Here's how the part is built. I have some questions about the finished solid (model axes, mm). A direction names the side the tool comes from. Round coordinates to 2 decimals unless told otherwise and drop trailing zeros. Order: outer loops, then holes, each group sorted by start corner. A loop starts at its lowest first (then second) coordinate and runs counter-clockwise, first axis right, second up. Notation, with made-up numbers: M 55,5.25 L 62,5.25 A18 ccw 62,23.25 Z; hole C 24.25,4 d8. An arc over 180 degrees is marked long. Use one line per item in the form item = value. Start each with the question number.
```python
from build123d import *

# Parameters (mm, degrees)
SKETCH1_W           = 10
SKETCH1_H           = 12
SKETCH1_R           = 0.7
BOSS_EXTRUDE1_DEPTH = 9
BOSS_EXTRUDE2_DEPTH = 10
BOSS_EXTRUDE4_DEPTH = 0.7
BOSS_EXTRUDE5_DEPTH = 10
FILLET1_R           = 1
FILLET2_R           = 0.25


with BuildPart() as part:
    # Sketch1 → Boss-Extrude1 (new body)
    # profile 1 of 3: a face of its own
    with BuildSketch(Plane.XY):
        Rectangle(SKETCH1_W, SKETCH1_H)
        with Locations((0, 4.5)):
            Circle(SKETCH1_R, mode=Mode.SUBTRACT)
        with Locations((0, -4.5)):
            Circle(SKETCH1_R, mode=Mode.SUBTRACT)
    # profile 2 of 3: a face of its own
    with BuildSketch(Plane.XY):
        with Locations((0, -4.5)):
            Circle(SKETCH1_R)
    # profile 3 of 3: a face of its own
    with BuildSketch(Plane.XY):
        with Locations((0, 4.5)):
            Circle(SKETCH1_R)
    extrude(amount=-BOSS_EXTRUDE1_DEPTH)

    # Sketch2 → Boss-Extrude2 (add)
    with BuildSketch(Plane(origin=(5, 0, 0), x_dir=(0, 0, -1), z_dir=(1, 0, 0))):
        with BuildLine():
            Line((3.4, 5.949159605), (0, 4.043822449))
            Line((0, 4.043822449), (0, -4.043822449))
            Line((0, -4.043822449), (3.4, -5.949159605))
            ThreePointArc((3.4, -5.949159605), (3.561551285, -5.976772876), (3.723791265, -6))
            Line((3.723791265, -6), (5.276208735, -6))
            ThreePointArc((5.276208735, -6), (5.438448715, -5.976772876), (5.6, -5.949159605))
            Line((5.6, -5.949159605), (9, -4.043822449))
            Line((9, -4.043822449), (9, 4.043822449))
            Line((9, 4.043822449), (5.6, 5.949159605))
            ThreePointArc((5.6, 5.949159605), (5.438448715, 5.976772876), (5.276208735, 6))
            Line((5.276208735, 6), (3.723791265, 6))
            ThreePointArc((3.723791265, 6), (3.561551285, 5.976772876), (3.4, 5.949159605))
        make_face()
        with BuildLine():
            ThreePointArc((5.276208735, 6), (4.5, 6.05), (3.723791265, 6))
            Line((3.723791265, 6), (5.276208735, 6))
        make_face()
        with BuildLine():
            Line((5.276208735, -6), (3.723791265, -6))
            ThreePointArc((3.723791265, -6), (4.5, -6.05), (5.276208735, -6))
        make_face()
    extrude(amount=BOSS_EXTRUDE2_DEPTH)

    # Sketch4 → Boss-Extrude4 (add)
    with BuildSketch(Plane.ZY.offset(5)):
        with BuildLine():
            ThreePointArc((-6.5, 0), (-4.5, -2), (-2.5, 0))
            Line((-2.5, 0), (-3, 0))
            ThreePointArc((-3, 0), (-4.5, -1.5), (-6, 0))
            Line((-6, 0), (-6.5, 0))
        make_face()
        with BuildLine():
            Line((-3, 0), (-2.5, 0))
            ThreePointArc((-2.5, 0), (-4.5, 2), (-6.5, 0))
            Line((-6.5, 0), (-6, 0))
            ThreePointArc((-6, 0), (-5.821691018, 0.709318583), (-5.329156198, 1.25))
            ThreePointArc((-5.329156198, 1.25), (-4.5, 1.5), (-3.670843802, 1.25))
            ThreePointArc((-3.670843802, 1.25), (-3.178308982, 0.709318583), (-3, 0))
        make_face()
        with BuildLine():
            ThreePointArc((-6.5, 0), (-4.5, -2), (-2.5, 0))
            Line((-2.5, 0), (-3, 0))
            ThreePointArc((-3, 0), (-4.5, -1.5), (-6, 0))
            Line((-6, 0), (-6.5, 0))
        make_face()
        with BuildLine():
            Line((-3, 0), (-2.5, 0))
            ThreePointArc((-2.5, 0), (-4.5, 2), (-6.5, 0))
            Line((-6.5, 0), (-6, 0))
            ThreePointArc((-6, 0), (-5.821691018, 0.709318583), (-5.329156198, 1.25))
            ThreePointArc((-5.329156198, 1.25), (-4.5, 1.5), (-3.670843802, 1.25))
            ThreePointArc((-3.670843802, 1.25), (-3.178308982, 0.709318583), (-3, 0))
        make_face()
        with BuildLine():
            Line((-6, 0), (-3, 0))
            ThreePointArc((-3, 0), (-3.178308982, 0.709318583), (-3.670843802, 1.25))
            Line((-3.670843802, 1.25), (-5.329156198, 1.25))
            ThreePointArc((-5.329156198, 1.25), (-5.821691018, 0.709318583), (-6, 0))
        make_face()
        with BuildLine():
            Line((-5.329156198, 1.25), (-3.670843802, 1.25))
            ThreePointArc((-3.670843802, 1.25), (-4.5, 1.5), (-5.329156198, 1.25))
        make_face()
        with BuildLine():
            ThreePointArc((-6, 0), (-4.5, -1.5), (-3, 0))
            Line((-3, 0), (-6, 0))
        make_face()
    extrude(amount=BOSS_EXTRUDE4_DEPTH)

    # Sketch4<3> → Boss-Extrude5 (add)
    with BuildSketch(Plane.ZY.offset(5)):
        with BuildLine():
            Line((-6, 0), (-3, 0))
            ThreePointArc((-3, 0), (-3.178308982, 0.709318583), (-3.670843802, 1.25))
            Line((-3.670843802, 1.25), (-5.329156198, 1.25))
            ThreePointArc((-5.329156198, 1.25), (-5.821691018, 0.709318583), (-6, 0))
        make_face()
        with BuildLine():
            ThreePointArc((-6, 0), (-4.5, -1.5), (-3, 0))
            Line((-3, 0), (-6, 0))
        make_face()
    extrude(amount=BOSS_EXTRUDE5_DEPTH)

    # Fillet1
    fillet1_edges = [part.edges().sort_by_distance(p)[0] for p in [
        (0, 6, -9),
        (0, -6, -9),
        (0, 6, 0),
        (0, -6, 0),
    ]]
    fillet(fillet1_edges, radius=FILLET1_R)

    # Fillet2
    fillet2_edges = [part.edges().sort_by_distance(p)[0] for p in [
        (-15, -1.321691018, -5.209318583),
    ]]
    fillet(fillet2_edges, radius=FILLET2_R - 0.0001)  # a hair under: the kernel refuses the full size


solid = part.part
```
1) If we section it at B-B on y = 3: Write out the boundary of the cut face in (x, z).
2) If we section it at A-A on x = 3.5: Write out the boundary of the cut face in (y, z).
3) On a 3-axis mill with a long thin cutter (end or side, diameter ignored), from which of +Z, -Z, +X, -X, +Y, -Y can I reach the whole of each face in a straight line? I mean faces 1 (the flat face through (9.93, -5.01, -7.276)), 2 (the flat face through (9.93, -4.983, -1.676)), 3 (the flat face through (-10, 1.25, -4)), 4 (the flat face through (-5.7, 1, -3)), 5 (the flat face through (5, 5, -1)). Say none if no direction works.
4) If we section it at C-C on x = -11: Write out the boundary of the cut face in (y, z), then the cut area to 3 significant figures.
5) Will these pins go through, and if not, where does the flat tip stop? pin 1 Ø0.5 at (x, z) = (-10, -5) entering from +Y; pin 2 Ø3 at (x, z) = (-2, -6.5) entering from +Y.
6) If I drill on line 1 (Y direction, x = -4.5, z = -6); line 2 (X direction, y = -0.25, z = -7); line 3 (Z direction, x = -12.5, y = -1.25), over which ranges is the centre line in solid material (lowest first)?
Completed:
q1.outline = M -5,-9 L 15,-9 L 15,0 L -5,0 Z
q2.outline = M -6,-8 A1 ccw -5,-9 L 5,-9 A1 ccw 6,-8 L 6,-1 A1 ccw 5,0 L -5,0 A1 ccw -6,-1 Z
q3.face_1 = -Z, +X, -Y
q3.face_2 = +Z, +X, -Y
q3.face_3 = +Z, -Z, -X, +Y
q3.face_4 = -X
q3.face_5 = +Z, +X, +Y
q4.outline = M 1.25,-5.33 L 1.25,-3.67 A1.5 ccw long Z
q4.area = 6.79 mm²
q5.pin_1 = 1.25
q5.pin_2 = 6
q6.line_1 = -6 to 6
q6.line_2 = -5 to 15
q6.line_3 = -5.33 to -3.67
